Source: CAD feature listing. Evaluate the final solid. Frame: model axes, mm. Face numbers are marked on the shaded views. A direction names the side the tool comes from. Round coordinates to 2 decimals unless told otherwise and drop trailing zeros. Write each loop counter-clockwise with the first axis right and the second up, starting at its lowest first coordinate (ties: lowest second). Pieces come first, ordered by that corner, then holes.
from build123d import *

# Parameters (mm, degrees)
F0_W      = 100
F0_H      = 100
F1_DEPTH  = 100
F2_W      = 20
F2_H      = 10
F3_DEPTH  = 10
F4_R      = 5
F5_DEPTH  = 100.001
F7_DEPTH  = 100.001
F9_DEPTH  = 25
F11_DEPTH = 25
F12_R     = 10
F13_SIZE  = 5


with BuildPart() as f1:
    # F0 (on Top) → F1 (new body)
    with BuildSketch(Plane.XY):
        with Locations((50, 50)):
            Rectangle(F0_W, F0_H)
    extrude(amount=F1_DEPTH)

    # F2 (on face) → F3 (cut)
    with BuildSketch(Plane.YZ.offset(100)):
        with Locations((50, 15)):
            Rectangle(F2_W, F2_H)
    extrude(amount=-F3_DEPTH, mode=Mode.SUBTRACT)

    # F4 (on face) → F5 (cut, through all)
    with BuildSketch(Plane.XY.offset(100)):
        with Locations((15, 75)):
            Circle(F4_R)
        with Locations((15, 50)):
            Circle(F4_R)
        with Locations((15, 25)):
            Circle(F4_R)
    extrude(amount=-F5_DEPTH, mode=Mode.SUBTRACT)

    # F6 (on face) → F7 (cut, through all)
    with BuildSketch(Plane.XZ):
        Polygon((100, 30), (100, 100), (30, 100), align=None)
    extrude(amount=-F7_DEPTH, mode=Mode.SUBTRACT)

    # F8 (on face) → F9 (cut)
    with BuildSketch(Plane.XZ):
        Polygon((100, 30), (30, 100), (30, 30), align=None)
    extrude(amount=-F9_DEPTH, mode=Mode.SUBTRACT)

    # F10 (on face) → F11 (cut)
    with BuildSketch(Plane(origin=(0, 100, 0), x_dir=(-1, 0, 0), z_dir=(0, 1, 0))):
        Polygon((-30, 100), (-100, 30), (-30, 30), align=None)
    extrude(amount=-F11_DEPTH, mode=Mode.SUBTRACT)

    # F12
    f12_edges = [f1.edges().sort_by_distance(p)[0] for p in [
        (30, 12.5, 30),
        (30, 87.5, 30),
    ]]
    fillet(f12_edges, radius=F12_R)

    # F13
    f13_edges = [f1.edges().sort_by_distance(p)[0] for p in [
        (100, 0, 15),
        (100, 100, 15),
    ]]
    chamfer(f13_edges, length=F13_SIZE)


solid = f1.part
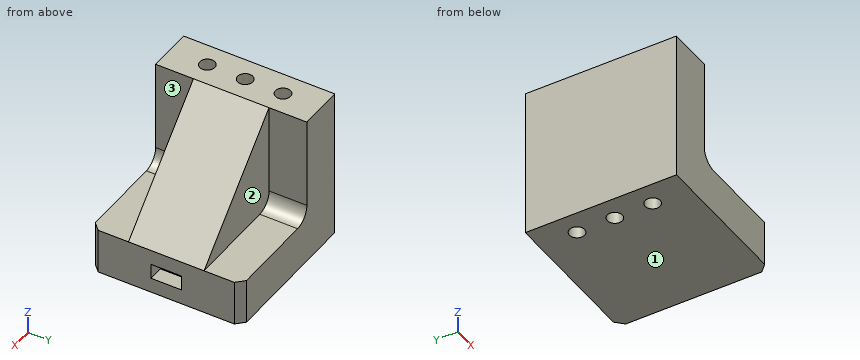
1) Contact query for flat-ended pins moving along their axis: P1, Ø1.5, axis at x = 89, y = 39.5, coming from the -Z side; P2, Ø6, axis at x = 82.5, y = 43.5, coming from the +Z side; P3, Ø7.5, axis at y = 17.5, z = 64.5, coming from the +X side; P4, Ø12.5, axis at x = 75.5, y = 10.5, coming from the +Z side. Output: stop coordinate, or through.
Taken from the geometry:
P1: stops at z = 0
P2: stops at z = 50.5
P3: stops at x = 30
P4: stops at z = 30
2) Section query D-D on y = 89. Return the cut outline in (x, z), then the cut area to 3 significant figures.
Taken from the geometry:
outline: (0, 0) - (100, 0) - (100, 30) - (40, 30) arc R10 cw to (30, 40) - (30, 100) - (0, 100) - close
area: 5,120 mm2
3) Section query C-C on y = 52. Return the cut outline in (x, z).
Taken from the geometry:
outline: (0, 0) - (10.42, 0) - (10.42, 100) - (0, 100) - close; (19.58, 0) - (100, 0) - (100, 10) - (90, 10) - (90, 20) - (100, 20) - (100, 30) - (30, 100) - (19.58, 100) - close
4) Reachability of the marked faces 1, 2 and 3 from +Z, -Z, +X, -X, +Y, -Y: full face, straight path, thin tool, end or side. Return the list, or none.
Taken from the geometry:
face 1: -Z, +X, -X, +Y, -Y
face 2: +Z, +X, +Y
face 3: +Z, +X, -Y
5) Section query A-A on z = 78. Return the cut outline in (x, y), then the cut area to 3 significant figures.
Taken from the geometry:
outline: (0, 0) - (30, 0) - (30, 25) - (52, 25) - (52, 75) - (30, 75) - (30, 100) - (0, 100) - close; hole circle Ø10 at (15, 25); hole circle Ø10 at (15, 50); hole circle Ø10 at (15, 75)
area: 3,860 mm2
6) Material intervals for line 1 (Y direction, x = 15, z = 36); line 2 (X direction, y = 50.5, z = 19); line 3 (Y direction, x = 10.5, z = 69), sorted ascending.
Taken from the geometry:
line 1: y = 0 to 20, 30 to 45, 55 to 70, 80 to 100
line 2: x = 0 to 10.03, 19.97 to 90
line 3: y = 0 to 22.82, 27.18 to 47.82, 52.18 to 72.82, 77.18 to 100
7) Section query B-B on x = 15. Return the cut outline in (y, z), then the cut area to 3 significant figures.
Taken from the geometry:
outline: (0, 0) - (20, 0) - (20, 100) - (0, 100) - close; (30, 0) - (45, 0) - (45, 100) - (30, 100) - close; (55, 0) - (70, 0) - (70, 100) - (55, 100) - close; (80, 0) - (100, 0) - (100, 100) - (80, 100) - close
area: 7,000 mm2
